Work out the finished part from the listing and answer in its coordinate system (mm). Face numbers are marked on the shaded views. A direction names the side the tool comes from. Coordinates: 2 decimals unless noted, no trailing zeros. Order: outer loops, then holes, each group sorted by start corner. A loop starts at its lowest first (then second) coordinate and runs counter-clockwise, first axis right, second up.
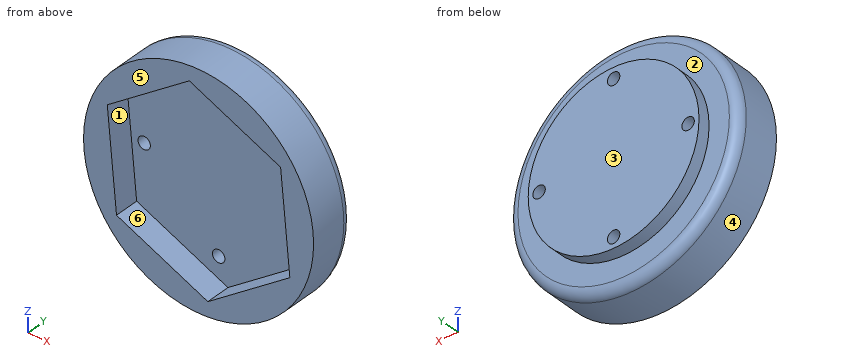
```python
from build123d import *

# Parameters (mm, degrees)
SKETCH2_R           = 27.469
BOSS_EXTRUDE1_DEPTH = 4
SKETCH3_R           = 2
CUT_EXTRUDE1_DEPTH  = 5
SKETCH4_R           = 37
BOSS_EXTRUDE2_DEPTH = 15
CUT_EXTRUDE3_DEPTH  = 8
FILLET1_R           = 3
SKETCH7_R           = 2
CUT_EXTRUDE5_DEPTH  = 25


with BuildPart() as part:
    # Sketch2 → Boss-Extrude1 (new body)
    with BuildSketch(Plane(origin=(0, 0, 0), x_dir=(1, 0, 0), z_dir=(0, 1, 0))):
        Circle(SKETCH2_R)
    extrude(amount=BOSS_EXTRUDE1_DEPTH)

    # Sketch3 → Cut-Extrude1 (cut, through all)
    with BuildSketch(Plane(origin=(0, 4, 0), x_dir=(1, 0, 0), z_dir=(0, 1, 0))):
        with Locations((-23.971, 0)):
            Circle(SKETCH3_R)
        with Locations((0, 23.971)):
            Circle(SKETCH3_R)
        with Locations((23.971, 0)):
            Circle(SKETCH3_R)
        with Locations((0, -23.971)):
            Circle(SKETCH3_R)
    extrude(amount=-CUT_EXTRUDE1_DEPTH, mode=Mode.SUBTRACT)

    # Sketch4 → Boss-Extrude2 (add)
    with BuildSketch(Plane.XZ):
        Circle(SKETCH4_R)
    extrude(amount=BOSS_EXTRUDE2_DEPTH)

    # Sketch6 → Cut-Extrude3 (cut)
    with BuildSketch(Plane.XZ.offset(15)):
        Polygon((-29.369836479, 13.518359314), (-26.392160823, -18.675844839), (2.977675656, -32.194204153), (29.369836479, -13.518359314), (26.392160823, 18.675844839), (-2.977675656, 32.194204153), align=None)
    extrude(amount=-CUT_EXTRUDE3_DEPTH, mode=Mode.SUBTRACT)

    # Fillet1
    fillet1_edges = [part.edges().sort_by_distance(p)[0] for p in [
        (-37, 0, 0),
    ]]
    fillet(fillet1_edges, radius=FILLET1_R)

    # Sketch7 → Cut-Extrude5 (cut, through all)
    with BuildSketch(Plane(origin=(0, 9, 0), x_dir=(1, 0, 0), z_dir=(0, 1, 0))):
        with Locations((0, 23.971)):
            Circle(SKETCH7_R)
        with Locations((23.971, 0)):
            Circle(SKETCH7_R)
        with Locations((0, -23.971)):
            Circle(SKETCH7_R)
        with Locations((-23.971, 0)):
            Circle(SKETCH7_R)
    extrude(amount=-CUT_EXTRUDE5_DEPTH, mode=Mode.SUBTRACT)


solid = part.part
```
1. Flat-ended cylindrical pins translate along their axes: pin 1 (8 mm diameter, centred on x = 24, z = -4, fed in from -Y); pin 2 (10 mm diameter, centred on x = -4, y = -8.5, fed in from -Z); pin 3 (8 mm diameter, centred on x = -25, y = -3.5, fed in from -Z); pin 4 (3 mm diameter, centred on x = 23.971, z = 0, fed in from -Y). Find the tip coordinate at first contact, or state that the pin passes through.
2. For the marked faces 1, 2 and 3, determine the directions among +Z, -Z, +X, -X, +Y, -Y from which every point of the face is accessible in a straight line to the end or side of a thin tool.
3. The part is cut by section B-B (x = 0). Determine the outline of the cut face in (y, z), plus the area to 3 significant figures.
4. The mould has two halves that part along Z. Classify the marked faces 4, 5 and 6: released by +Z, released by -Z, zero draft, split by the parting line, or undercut.
5. Consider probe 1 along Z at (x, y) = (0, -5.75); probe 2 along Z at (x, y) = (0, 0.25); probe 3 along Y at (x, z) = (-8.5, 16.5). Determine where each line is inside the solid, lowest interval first.
6. The part is cut by section C-C (y = -5.75). Determine the outline of the cut face in (x, z), plus the area to 3 significant figures.
7. The part is cut by section A-A (y = -12). Determine the outline of the cut face in (x, z).
Worked out:
1. pin 1: stops at y = -7
1. pin 2: stops at z = -37
1. pin 3: stops at z = -30.46
1. pin 4: passes through
2. face 1: -Y
2. face 2: +Y
2. face 3: +Z, -Z, +X, -X, +Y
3. outline: (-15, -37) - (-3, -37) arc R3 ccw to (0, -34) - (0, -27.47) - (4, -27.47) - (4, -25.97) - (-7, -25.97) - (-7, -30.82) - (-15, -30.82) - close; (-15, 30.82) - (-7, 30.82) - (-7, 25.97) - (4, 25.97) - (4, 27.47) - (0, 27.47) - (0, 34) arc R3 ccw to (-3, 37) - (-15, 37) - close; (-7, -21.97) - (4, -21.97) - (4, 21.97) - (-7, 21.97) - close
3. area: 745 mm2
4. face 4: split by the parting line
4. face 5: zero draft
4. face 6: undercut
5. probe 1: z = -37 to -25.97, -21.97 to 21.97, 25.97 to 37
5. probe 2: z = -27.47 to -25.97, -21.97 to 21.97, 25.97 to 27.47
5. probe 3: y = -7 to 4
6. outline: circle Ø74 at (0, 0); hole circle Ø4 at (-23.97, 0); hole circle Ø4 at (0, -23.97); hole circle Ø4 at (0, 23.97); hole circle Ø4 at (23.97, 0)
6. area: 4,250 mm2
7. outline: circle Ø74 at (0, 0); hole (-29.37, 13.52) - (-26.39, -18.68) - (2.98, -32.19) - (29.37, -13.52) - (26.39, 18.68) - (-2.98, 32.19) - close
